from build123d import *

# Parameters (mm, degrees)
F1_DEPTH = 53
F2_W     = 5
F2_H     = 33
F3_DEPTH = 19
F4_R     = 3.5
F5_DEPTH = 5
F0_R     = 1.6
F6_DEPTH = 4
F7_R     = 2
F8_DEPTH = 50
F9_R     = 1


with BuildPart() as f1:
    # F0 (on Top) → F1 (new body)
    with BuildSketch(Plane.XY):
        Polygon((19, 4), (19, 16.5), (8, 16.5), (8, 20.5), (0, 20.5), (-8, 20.5), (-8, 16.5), (-19, 16.5), (-19, 4), (-19, -4), (-19, -16.5), (19, -16.5), (19, -4), align=None)
    extrude(amount=F1_DEPTH)

    # F2 (on face) → F3 (cut)
    with BuildSketch(Plane.XY.offset(53)):
        with Locations((-16.5, 0)):
            Rectangle(F2_W, F2_H)
        with Locations((16.5, 0)):
            Rectangle(F2_W, F2_H)
    extrude(amount=-F3_DEPTH, mode=Mode.SUBTRACT)

    # F4 (on face) → F5 (cut)
    with BuildSketch(Plane(origin=(0, 20.5, 0), x_dir=(-1, 0, 0), z_dir=(0, 1, 0))):
        with Locations((0, 30)):
            Circle(F4_R)
    extrude(amount=-F5_DEPTH, mode=Mode.SUBTRACT)

    # F0 (on Top) → F6 (join)
    with BuildSketch(Plane.XY):
        with BuildLine():
            Line((-23, -4), (-19, -4))
            Line((-19, -4), (-19, 4))
            Line((-19, 4), (-23, 4))
            ThreePointArc((-23, 4), (-27, 0), (-23, -4))
        make_face()
        with Locations((-23, 0)):
            Circle(F0_R, mode=Mode.SUBTRACT)
        with BuildLine():
            Line((23, 4), (19, 4))
            Line((19, 4), (19, -4))
            Line((19, -4), (23, -4))
            ThreePointArc((23, -4), (27, 0), (23, 4))
        make_face()
        with Locations((23, 0)):
            Circle(F0_R, mode=Mode.SUBTRACT)
    extrude(amount=F6_DEPTH)

    # F7 (on face) → F8 (join)
    with BuildSketch(Plane(origin=(0, 15.5, 0), x_dir=(-1, 0, 0), z_dir=(0, 1, 0))):
        with Locations((0, 30)):
            Circle(F7_R)
    extrude(amount=F8_DEPTH)

    # F9
    f9_edges = [f1.edges().sort_by_distance(p)[0] for p in [
        (14, 0, 53),
        (0, -16.5, 53),
        (-14, 0, 53),
        (-11, 16.5, 53),
        (-8, 18.5, 53),
        (0, 20.5, 53),
        (8, 18.5, 53),
        (11, 16.5, 53),
        (-14, -16.5, 43.5),
        (-14, 16.5, 43.5),
        (-14, 0, 34),
        (14, 16.5, 43.5),
        (14, -16.5, 43.5),
        (14, 0, 34),
        (-19, -16.5, 17),
        (-16.5, -16.5, 34),
        (16.5, -16.5, 34),
        (19, -16.5, 17),
        (19, 0, 34),
        (19, 16.5, 17),
        (19, 0, 4),
        (19, -4, 2),
        (19, 4, 2),
        (8, 16.5, 26.5),
        (8, 20.5, 26.5),
        (-8, 20.5, 26.5),
        (-19, 16.5, 17),
        (-8, 16.5, 26.5),
        (-19, 0, 34),
        (-19, 4, 2),
        (-19, 0, 4),
        (-19, -4, 2),
        (16.5, 16.5, 34),
        (-16.5, 16.5, 34),
    ]]
    fillet(f9_edges, radius=F9_R)


solid = f1.part
CAD build for the part. Positions are in the model's coordinates, mm. A direction names the side the tool comes from. Round coordinates to 2 decimals unless told otherwise and drop trailing zeros. Order: outer loops, then holes, each group sorted by start corner. A loop starts at its lowest first (then second) coordinate and runs counter-clockwise, first axis right, second up. Notation, with made-up numbers: (50, 89.5) -> (98, 89.5) arc R15 cw to (98, 112.5) -> close; hole circle Ø1 at (83.25, -27.75). An arc over 180 degrees is marked (long way). Write each question's results on one line, items separated by ' | '.
1. Wall check: line 1 along Y through (x, z) = (-23, 3.2); line 2 along Z through (x, y) = (0, 19); line 3 along Y through (x, z) = (-5.5, 8.5). Give the ranges that are in metal, low to high. Write a range as [from, to].
Findings below:
line 1: y = [-4, -1.6], [1.6, 4] | line 2: z = [0, 26.5], [28, 32], [33.5, 53] | line 3: y = [-16.5, 20.5]
2. Cut at D-D (y = 9.5). Give the cut face in (x, z), plus the area to 3 significant figures.
Findings below:
outline: (-19, 0) -> (19, 0) -> (19, 33) arc R1 ccw to (18, 34) -> (15, 34) arc R1 cw to (14, 35) -> (14, 52) arc R1 ccw to (13, 53) -> (-13, 53) arc R1 ccw to (-14, 52) -> (-14, 35) arc R1 cw to (-15, 34) -> (-18, 34) arc R1 ccw to (-19, 33) -> close | area: 1,820 mm²
3. Cut at A-A (y = 0). Give the cut face in (x, z), plus the area to 3 significant figures.
Findings below:
outline: (-27, 0) -> (-24.6, 0) -> (-24.6, 4) -> (-27, 4) -> close; (-21.4, 0) -> (21.4, 0) -> (21.4, 4) -> (20, 4) arc R1 cw to (19, 5) -> (19, 33) arc R1 ccw to (18, 34) -> (15, 34) arc R1 cw to (14, 35) -> (14, 52) arc R1 ccw to (13, 53) -> (-13, 53) arc R1 ccw to (-14, 52) -> (-14, 35) arc R1 cw to (-15, 34) -> (-18, 34) arc R1 ccw to (-19, 33) -> (-19, 5) arc R1 cw to (-20, 4) -> (-21.4, 4) -> close; (24.6, 0) -> (27, 0) -> (27, 4) -> (24.6, 4) -> close | area: 1,860 mm²
4. Cut at C-C (z = 30). Give the cut face in (x, y), plus the area to 3 significant figures.
Findings below:
outline: (-19, -15.5) arc R1 ccw to (-18, -16.5) -> (18, -16.5) arc R1 ccw to (19, -15.5) -> (19, 15.5) arc R1 ccw to (18, 16.5) -> (9, 16.5) arc R1 cw to (8, 17.5) -> (8, 19.5) arc R1 ccw to (7, 20.5) -> (3.5, 20.5) -> (3.5, 15.5) -> (2, 15.5) -> (2, 65.5) -> (-2, 65.5) -> (-2, 15.5) -> (-3.5, 15.5) -> (-3.5, 20.5) -> (-7, 20.5) arc R1 ccw to (-8, 19.5) -> (-8, 17.5) arc R1 cw to (-9, 16.5) -> (-18, 16.5) arc R1 ccw to (-19, 15.5) -> close | area: 1,480 mm²
5. Cut at B-B (x = -16). Give the cut face in (y, z), plus the area to 3 significant figures.
Findings below:
outline: (-16.5, 0) -> (16.5, 0) -> (16.5, 33) arc R1 ccw to (15.5, 34) -> (-15.5, 34) arc R1 ccw to (-16.5, 33) -> close | area: 1,120 mm²
6. Flat gauge pins, fed straight in: P1, Ø1, axis at y = 19, z = 17, coming from the -X side; P2, Ø1.5, axis at x = -8, z = 21, coming from the +Y side; P3, Ø3.5, axis at x = 17, y = -2.5, coming from the +Z side. Where does each tip first touch, or does it go through?
Findings below:
P1: stops at x = -8 | P2: stops at y = 20.47 | P3: stops at z = 34
7. 3-axis set-ups, long thin cutter, end or side, ignore diameter. For faces 1 (the face through (-22, -4, 2)), 2 (the face through (-2, 15.5, 28)), 3 (the face through (-13, 16.5, 20)): which of +Z, -Z, +X, -X, +Y, -Y reach the whole face in a straight line?
Findings below:
face 1: +Z, -Z, -X, -Y | face 2: +Y | face 3: +Z, -Z, -X, +Y
8. Pull direction X, two halves, no side cores. Call faces 4 (the face through (24.526, 0.481, 1.972)), 5 (the face through (14, 0, 44)), 6 (the face through (-14, 0, 44)), 7 (the face through (21, -4, 2)): pulls with the +X half, pulls with the -X half, needs draft (parallel to the pull), parting line crosses it, or undercut.
Findings below:
face 4: undercut | face 5: pulls with the +X half | face 6: pulls with the -X half | face 7: needs draft
